Read the model definition and answer for the solid it produces. Units are mm, in the model's axes. Coordinates: 2 decimals unless noted, no trailing zeros. Loops run counter-clockwise (first coordinate to the right, second up) from the corner with the lowest first, then second, coordinate; pieces in that order, holes last. Notation, with made-up numbers: (-2.5, 30.25) -> (19.5, 30.25) arc R15 cw to (19.5, 57.25) -> close; hole circle Ø1 at (58, 21.25). An arc over 180 degrees is marked (long way). One line per question, with ' | ' between items. Start each with the question number.
Solid Edge part; units mm, degrees
sketch "Sketch1" plane through (0, 0, 0) normal (0, -1, 0) x (1, 0, 0)
  line L0 (-22.5, -72.5) -> (22.5, -72.5)
  line L1 (22.5, -72.5) -> (22.5, 72.5)
  line L2 (22.5, 72.5) -> (-22.5, 72.5)
  line L3 (-22.5, 72.5) -> (-22.5, -72.5)
extrude "Protrusion1" add sketch "Sketch1" against normal blind 2370
sketch "Sketch2" plane through (22.5, 1185, 0) normal (1, 0, 0) x (0, 1, 0)
  line L0 (1035, 72.5) -> (1035, 36.25)
  line L1 (1035, 36.25) -> (990, 36.25)
  line L2 (990, 36.25) -> (990, 72.5)
  line L3 (990, 72.5) -> (1035, 72.5)
  line L4 (-1035, 72.5) -> (-1035, 36.25)
  line L5 (-1035, 36.25) -> (-990, 36.25)
  line L6 (-990, 36.25) -> (-990, 72.5)
  line L7 (-990, 72.5) -> (-1035, 72.5)
extrude "ExtrudedCutout_1" cut sketch "Sketch2" against normal blind 89.2118
mirror "Mirror1" about plane through (0, 0, 0) normal (0, 0, -1) of "ExtrudedCutout_1"
sketch "Sketch3" plane through (22.5, 1185, 0) normal (1, 0, 0) x (0, 1, 0)
  line L0 (990, 145) -> (-1185, -166.4815)
  line L1 (-1185, -166.4815) -> (-1185, 145)
  line L2 (-1185, 145) -> (990, 145)
extrude "ExtrudedCutout_3" cut sketch "Sketch3" against normal blind 53.381
properties material "Wood, Pine"
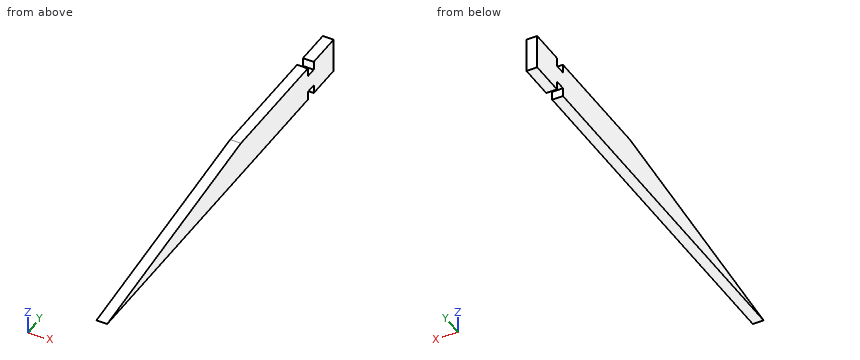
(1) Find the intervals of material crossed by probe 1 along Z at (x, y) = (-4, 2188.5); probe 2 along Z at (x, y) = (-8.5, 1038), in increasing order. Write a range as from..to.
(2) Section B-B on x = 11 is taken. Write down the section's boundary in (y, z), plus the area to 3 significant figures.
(3) Section C-C on y = 1587.5 is taken. Write down the section's boundary in (x, z), plus the area to 3 significant figures.
(4) This flat-tipped pin is pushed along its axis until it touches: pin 1 Ø13.5 at (x, y) = (5.5, 2193.5) entering from +Z. Where does it stop, or does it pass through?
(5) Section A-A on z = 51.5 is taken. Write down the section's boundary in (x, y).
Working result:
1) probe 1: z = -36.25..36.25 | probe 2: z = -72.5..-17.83
2) outline: (656.25, -72.5) -> (2175, -72.5) -> (2175, -36.25) -> (2220, -36.25) -> (2220, -72.5) -> (2370, -72.5) -> (2370, 72.5) -> (2220, 72.5) -> (2220, 36.25) -> (2175, 36.25) -> (2175, 72.5) -> (1668.75, 72.5) -> close | area: 172,000 mm2
3) outline: (-22.5, -72.5) -> (22.5, -72.5) -> (22.5, 60.86) -> (-22.5, 60.86) -> close | area: 6,000 mm2
4) pin 1: stops at z = 36.25
5) outline: (-22.5, 1522.11) -> (22.5, 1522.11) -> (22.5, 2175) -> (-22.5, 2175) -> close; (-22.5, 2220) -> (22.5, 2220) -> (22.5, 2370) -> (-22.5, 2370) -> close
